from build123d import *

# Parameters (mm, degrees)
SKETCH16_R          = 64.85
SKETCH16_R_2        = 2.5
SKETCH16_R_3        = 4.1275
BOSS_EXTRUDE1_DEPTH = 10


with BuildPart() as part:
    # Sketch16 → Boss-Extrude1 (new body)
    with BuildSketch(Plane.XZ.offset(-75)):
        with Locations(Location((0, 0, 0), (0, 0, 90))):
            Circle(SKETCH16_R)
        with Locations(Location((38.382245896, -22.16, 0), (0, 0, 90))):
            Circle(SKETCH16_R_2, mode=Mode.SUBTRACT)
        with Locations(Location((51.961524227, -30, 0), (0, 0, 90))):
            Circle(SKETCH16_R_2, mode=Mode.SUBTRACT)
        with Locations(Location((-43.132245896, -13.932758664, 0), (0, 0, 90))):
            Circle(SKETCH16_R_2, mode=Mode.SUBTRACT)
        with Locations(Location((-38.382245896, -22.16, 0), (0, 0, 90))):
            Circle(SKETCH16_R_2, mode=Mode.SUBTRACT)
        with Locations(Location((-51.961524227, -30, 0), (0, 0, 90))):
            Circle(SKETCH16_R_2, mode=Mode.SUBTRACT)
        with Locations(Location((0, 44.32, 0), (0, 0, 90))):
            Circle(SKETCH16_R_2, mode=Mode.SUBTRACT)
        with Locations(Location((0, 60, 0), (0, 0, 90))):
            Circle(SKETCH16_R_2, mode=Mode.SUBTRACT)
        with Locations(Location((-33.632245896, -30.387241336, 0), (0, 0, 90))):
            Circle(SKETCH16_R_2, mode=Mode.SUBTRACT)
        with Locations(Location((-47.211524227, -38.227241336, 0), (0, 0, 90))):
            Circle(SKETCH16_R_2, mode=Mode.SUBTRACT)
        with Locations(Location((-56.711524227, -21.772758664, 0), (0, 0, 90))):
            Circle(SKETCH16_R_2, mode=Mode.SUBTRACT)
        with Locations(Location((9.5, 44.32, 0), (0, 0, 90))):
            Circle(SKETCH16_R_2, mode=Mode.SUBTRACT)
        with Locations(Location((-9.5, 44.32, 0), (0, 0, 90))):
            Circle(SKETCH16_R_2, mode=Mode.SUBTRACT)
        with Locations(Location((-9.5, 60, 0), (0, 0, 90))):
            Circle(SKETCH16_R_2, mode=Mode.SUBTRACT)
        with Locations(Location((9.5, 60, 0), (0, 0, 90))):
            Circle(SKETCH16_R_2, mode=Mode.SUBTRACT)
        with Locations(Location((33.632245896, -30.387241336, 0), (0, 0, 90))):
            Circle(SKETCH16_R_2, mode=Mode.SUBTRACT)
        with Locations(Location((43.132245896, -13.932758664, 0), (0, 0, 90))):
            Circle(SKETCH16_R_2, mode=Mode.SUBTRACT)
        with Locations(Location((56.711524227, -21.772758664, 0), (0, 0, 90))):
            Circle(SKETCH16_R_2, mode=Mode.SUBTRACT)
        with Locations(Location((47.211524227, -38.227241336, 0), (0, 0, 90))):
            Circle(SKETCH16_R_2, mode=Mode.SUBTRACT)
        with Locations(Location((0, 0, 0), (0, 0, 90))):
            Circle(SKETCH16_R_3, mode=Mode.SUBTRACT)
    extrude(amount=BOSS_EXTRUDE1_DEPTH)


solid = part.part
Geometry check sheet. Reference: the model listing, model coordinates, mm. Give positions to 0.01 mm unless a question says otherwise; leave off trailing zeros. Order: outer loops, then holes, each group sorted by start corner. A loop starts at its lowest first (then second) coordinate and runs counter-clockwise, first axis right, second up. Notation, with made-up numbers: (77.5, 0.25) - (136.5, 0.25) arc R21 cw to (136.5, 4.25) - close; hole circle Ø10 at (69.25, -3.75). An arc over 180 degrees is marked (long way). Use one line per item in the form item = value.
1) Draft check along X on faces 1 (the face through (10.46, 70.07, 62.31)), 2 (the face through (14, 65, -1)). Enter one of: released by +X, released by -X, zero draft, split by the parting line, or undercut.
Working result:
face_1 = undercut
face_2 = zero draft
2) Depth check by flat-ended pin: pin 1 Ø6 at (x, z) = (-9.5, 44.32) entering from +Y; pin 2 Ø2 at (y, z) = (70, 1) entering from -X; pin 3 Ø3 at (x, z) = (-56.71, -21.77) entering from -Y; pin 4 Ø1 at (x, y) = (-21, 70) entering from +Z. Enter the tip coordinate at first touch or a pass-through.
Working result:
pin_1 = 75
pin_2 = -64.85
pin_3 = through
pin_4 = 61.52
3) Sectioned sample at A-A (x = 0). Record the boundary of the cut face in (y, z), and give its area (3 significant figures).
Working result:
outline = (65, -64.85) - (75, -64.85) - (75, -4.13) - (65, -4.13) - close; (65, 4.13) - (75, 4.13) - (75, 41.82) - (65, 41.82) - close; (65, 46.82) - (75, 46.82) - (75, 57.5) - (65, 57.5) - close; (65, 62.5) - (75, 62.5) - (75, 64.85) - (65, 64.85) - close
area = 1,110 mm^2
4) Sectioned sample at D-D (y = 70.5). Count the separate pieces of the cut face and the enclosed holes in it, and give its area (3 significant figures).
Working result:
separate_pieces = 1
enclosed_holes = 19
area = 12,800 mm^2
5) Sectioned sample at B-B (z = -22.16). Record the boundary of the cut face in (x, y), and give its area (3 significant figures).
Working result:
outline = (-60.95, 65) - (-59.18, 65) - (-59.18, 75) - (-60.95, 75) - close; (-54.24, 65) - (-40.88, 65) - (-40.88, 75) - (-54.24, 75) - close; (-35.88, 65) - (35.88, 65) - (35.88, 75) - (-35.88, 75) - close; (40.88, 65) - (54.24, 65) - (54.24, 75) - (40.88, 75) - close; (59.18, 65) - (60.95, 65) - (60.95, 75) - (59.18, 75) - close
area = 1,020 mm^2
6) Material ranges on probe 1 along X at (y, z) = (70.75, 0); probe 2 along Z at (x, y) = (47, 68); probe 3 along X at (y, z) = (72, -30), recorded low to high. Write a range as from..to.
Working result:
probe_1 = -64.85..-4.13, 4.13..64.85
probe_2 = -44.68..-40.72, -35.74..44.68
probe_3 = -57.49..-54.46, -49.46..-36.1, -31.16..31.16, 36.1..49.46, 54.46..57.49
7) Sectioned sample at C-C (z = 60). Record the boundary of the cut face in (x, y).
Working result:
outline = (-24.61, 65) - (-12, 65) - (-12, 75) - (-24.61, 75) - close; (-7, 65) - (-2.5, 65) - (-2.5, 75) - (-7, 75) - close; (2.5, 65) - (7, 65) - (7, 75) - (2.5, 75) - close; (12, 65) - (24.61, 65) - (24.61, 75) - (12, 75) - close
